```python
from build123d import *

# Parameters (mm, degrees)
BOSS_EXTRUDE1_DEPTH      = 6
SKETCH3_R                = 20.1
CUT_EXTRUDE1_DEPTH       = 6
M5_CLEARANCE_HOLE1_D     = 5.5
CUT_EXTRUDE2_DEPTH       = 6
CUT_EXTRUDE4_DEPTH       = 6
M5_CLEARANCE_HOLE3_D     = 5.5
M5_CLEARANCE_HOLE2_D     = 5.5
M5_CLEARANCE_HOLE2_DEPTH = 10
M5_CLEARANCE_HOLE2_TIP   = 1.652366702
SKETCH21_W               = 6.3
SKETCH21_H               = 1.5
CUT_EXTRUDE5_DEPTH       = 6
SKETCH22_W               = 6.3
SKETCH22_H               = 1.5
CUT_EXTRUDE6_DEPTH       = 10


with BuildPart() as part:
    # Sketch1 → Boss-Extrude1 (new body)
    with BuildSketch(Plane.XY):
        with BuildLine():
            Line((-55, -85), (55, -85))
            ThreePointArc((55, -85), (58.535533906, -83.535533906), (60, -80))
            Line((60, -80), (60, 80))
            ThreePointArc((60, 80), (58.535533906, 83.535533906), (55, 85))
            Line((55, 85), (-55, 85))
            ThreePointArc((-55, 85), (-58.535533906, 83.535533906), (-60, 80))
            Line((-60, 80), (-60, -80))
            ThreePointArc((-60, -80), (-58.535533906, -83.535533906), (-55, -85))
        make_face()
    extrude(amount=BOSS_EXTRUDE1_DEPTH)

    # Sketch3 → Cut-Extrude1 (cut)
    with BuildSketch(Plane.XY.offset(6)):
        with Locations((0, 45)):
            Circle(SKETCH3_R)
    extrude(amount=-CUT_EXTRUDE1_DEPTH, mode=Mode.SUBTRACT)

    # M5 Clearance Hole1 (through all)
    with Locations(Plane.XY.offset(6)):
        with Locations((-23.57, 68.57), (23.57, 68.57), (23.57, 21.43), (-23.57, 21.43)):
            Hole(M5_CLEARANCE_HOLE1_D / 2)

    # Sketch11 → Cut-Extrude2 (cut)
    with BuildSketch(Plane.XY.offset(6)):
        with BuildLine():
            Line((-42.82, 24.93), (-42.82, 17.93))
            ThreePointArc((-42.82, 17.93), (-45.57, 15.18), (-48.32, 17.93))
            Line((-48.32, 17.93), (-48.32, 24.93))
            ThreePointArc((-48.32, 24.93), (-45.57, 27.68), (-42.82, 24.93))
        make_face()
        with BuildLine():
            Line((42.82, 24.93), (42.82, 17.93))
            ThreePointArc((42.82, 17.93), (45.57, 15.18), (48.32, 17.93))
            Line((48.32, 17.93), (48.32, 24.93))
            ThreePointArc((48.32, 24.93), (45.57, 27.68), (42.82, 24.93))
        make_face()
    extrude(amount=-CUT_EXTRUDE2_DEPTH, mode=Mode.SUBTRACT)

    # Sketch15 → Cut-Extrude4 (cut)
    with BuildSketch(Plane.XY.offset(6)):
        with BuildLine():
            Line((-51.25, 47.75), (-46.25, 47.75))
            ThreePointArc((-46.25, 47.75), (-43.5, 45), (-46.25, 42.25))
            Line((-46.25, 42.25), (-51.25, 42.25))
            ThreePointArc((-51.25, 42.25), (-54, 45), (-51.25, 47.75))
        make_face()
        with BuildLine():
            Line((-51.25, 57.75), (-46.25, 57.75))
            ThreePointArc((-46.25, 57.75), (-43.5, 55), (-46.25, 52.25))
            Line((-46.25, 52.25), (-51.25, 52.25))
            ThreePointArc((-51.25, 52.25), (-54, 55), (-51.25, 57.75))
        make_face()
        with BuildLine():
            Line((51.25, 47.75), (46.25, 47.75))
            ThreePointArc((46.25, 47.75), (43.5, 45), (46.25, 42.25))
            Line((46.25, 42.25), (51.25, 42.25))
            ThreePointArc((51.25, 42.25), (54, 45), (51.25, 47.75))
        make_face()
        with BuildLine():
            Line((51.25, 57.75), (46.25, 57.75))
            ThreePointArc((46.25, 57.75), (43.5, 55), (46.25, 52.25))
            Line((46.25, 52.25), (51.25, 52.25))
            ThreePointArc((51.25, 52.25), (54, 55), (51.25, 57.75))
        make_face()
    extrude(amount=-CUT_EXTRUDE4_DEPTH, mode=Mode.SUBTRACT)

    # M5 Clearance Hole3 (through all)
    with Locations(Plane.XY.offset(6)):
        with Locations((-45.57, -39.97), (45.57, -39.97), (20, -73), (0, -73), (-20, -73)):
            Hole(M5_CLEARANCE_HOLE3_D / 2)

    # M5 Clearance Hole2
    with Locations(Plane(origin=(0, 0, 0), x_dir=(-1, 0, 0), z_dir=(0, 0, -1))):
        with Locations((0, -53)):
            Hole(M5_CLEARANCE_HOLE2_D / 2, depth=M5_CLEARANCE_HOLE2_DEPTH)
            with Locations((0, 0, -(M5_CLEARANCE_HOLE2_DEPTH + M5_CLEARANCE_HOLE2_TIP / 2))):  # 118° drill point
                Cone(0, M5_CLEARANCE_HOLE2_D / 2, M5_CLEARANCE_HOLE2_TIP, mode=Mode.SUBTRACT)

    # Sketch21 → Cut-Extrude5 (cut)
    with BuildSketch(Plane(origin=(0, 0, 0), x_dir=(-1, 0, 0), z_dir=(0, 0, -1))):
        with Locations((0, -47)):
            Rectangle(SKETCH21_W, SKETCH21_H)
    extrude(amount=-CUT_EXTRUDE5_DEPTH, mode=Mode.SUBTRACT)

    # Sketch22 → Cut-Extrude6 (cut)
    with BuildSketch(Plane.XY.offset(6)):
        with Locations((0, -63)):
            Rectangle(SKETCH22_W, SKETCH22_H)
    extrude(amount=-CUT_EXTRUDE6_DEPTH, mode=Mode.SUBTRACT)


solid = part.part
```
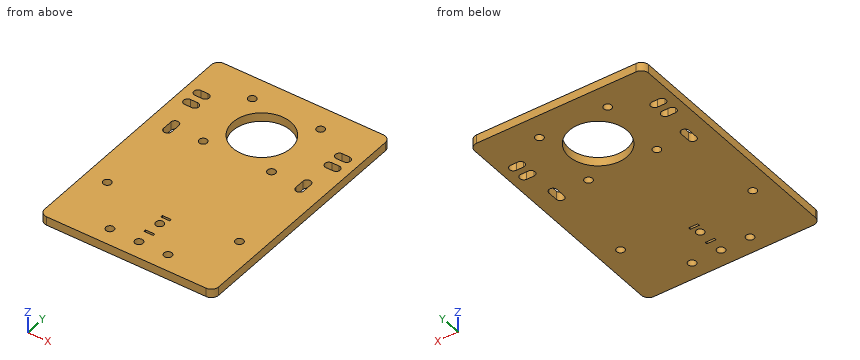
Design review of the part built by this model. Coordinates are the model's own, in mm. Coordinates: 2 decimals unless noted, no trailing zeros. Order: outer loops, then holes, each group sorted by start corner. A loop starts at its lowest first (then second) coordinate and runs counter-clockwise, first axis right, second up.
1) Take a section at B-B, the plane x = 0. Give the boundary of the cut face in (y, z).
2) Take a section at C-C, the plane z = 4.05. State how many separate pieces and enclosed holes the cut face has, and give its area (3 significant figures).
3) Take a section at A-A, the plane y = -39.97. Give the boundary of the cut face in (x, z), and give its area (3 significant figures).
4) Wall thickness on line 1 along Y through (x, z) = (23.57, 3.5); line 2 along Y through (x, z) = (0, 2.25); line 3 along Y through (x, z) = (-50.5, 1.35): over which ranges is each line inside the solid? List them lowest first.
Returned:
1. outline: (-85, 0) - (-75.75, 0) - (-75.75, 6) - (-85, 6) - close; (-70.25, 0) - (-63.75, 0) - (-63.75, 6) - (-70.25, 6) - close; (-62.25, 0) - (-55.75, 0) - (-55.75, 6) - (-62.25, 6) - close; (-50.25, 0) - (-47.75, 0) - (-47.75, 6) - (-50.25, 6) - close; (-46.25, 0) - (24.9, 0) - (24.9, 6) - (-46.25, 6) - close; (65.1, 0) - (85, 0) - (85, 6) - (65.1, 6) - close
2. separate pieces: 1
2. enclosed holes: 19
2. area: 18,500 mm2
3. outline: (-60, 0) - (-48.32, 0) - (-48.32, 6) - (-60, 6) - close; (-42.82, 0) - (42.82, 0) - (42.82, 6) - (-42.82, 6) - close; (48.32, 0) - (60, 0) - (60, 6) - (48.32, 6) - close
3. area: 654 mm2
4. line 1: y = -85 to 18.68, 24.18 to 65.82, 71.32 to 85
4. line 2: y = -85 to -75.75, -70.25 to -63.75, -62.25 to -55.75, -50.25 to -47.75, -46.25 to 24.9, 65.1 to 85
4. line 3: y = -85 to 42.25, 47.75 to 52.25, 57.75 to 85
